Input: part model. Units: mm. Frame: model coordinates. Coordinates: 2 decimals unless noted, no trailing zeros. Order: outer loops, then holes, each group sorted by start corner. A loop starts at its lowest first (then second) coordinate and runs counter-clockwise, first axis right, second up. Notation, with made-up numbers: (-32.75, -39) -> (17.25, -39) arc R13 ccw to (17.25, -29) -> close; hole circle Ø2 at (41.25, -7). An arc over 180 degrees is marked (long way). Answer as CSV lines item,"result".
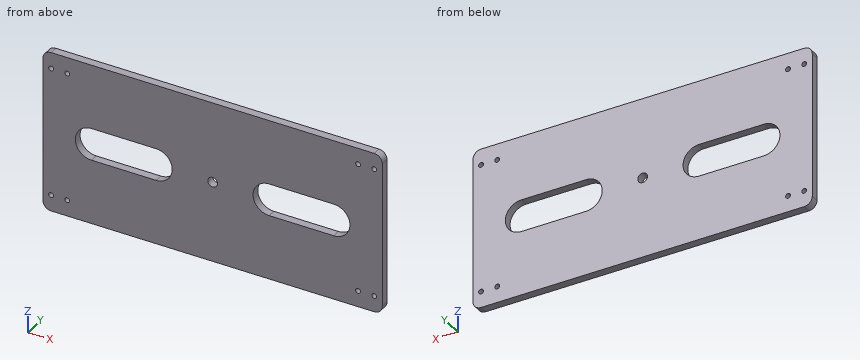
from build123d import *

# Parameters (mm, degrees)
SKETCH_1_W          = 210
SKETCH_1_H          = 100
EXTRUDE_1_DEPTH     = 5
CUT_EXTRUDE_1_DEPTH = 40
SKETCH_4_R          = 3
CUT_EXTRUDE_3_DEPTH = 20
SKETCH_8_R          = 1.5
CUT_EXTRUDE_4_DEPTH = 20
FILLET_1_R          = 5


with BuildPart() as part:
    # 草图1 → 凸台-拉伸1 (new body)
    with BuildSketch(Plane(origin=(0, 0, 0), x_dir=(1, 0, 0), z_dir=(0, 1, 0))):
        with Locations((105, -50)):
            Rectangle(SKETCH_1_W, SKETCH_1_H)
    extrude(amount=EXTRUDE_1_DEPTH)

    # 草图2 → 切除-拉伸1 (cut)
    with BuildSketch(Plane(origin=(0, 5, 0), x_dir=(1, 0, 0), z_dir=(0, 1, 0))):
        with BuildLine():
            Line((30, -40), (70, -40))
            ThreePointArc((70, -40), (80, -50), (70, -60))
            Line((70, -60), (30, -60))
            ThreePointArc((30, -60), (20, -50), (30, -40))
        make_face()
        with BuildLine():
            Line((140, -40), (180, -40))
            ThreePointArc((180, -40), (190, -50), (180, -60))
            Line((180, -60), (140, -60))
            ThreePointArc((140, -60), (130, -50), (140, -40))
        make_face()
    extrude(amount=-CUT_EXTRUDE_1_DEPTH, mode=Mode.SUBTRACT)

    # 草图4 → 切除-拉伸3 (cut)
    with BuildSketch(Plane(origin=(0, 5, 0), x_dir=(1, 0, 0), z_dir=(0, 1, 0))):
        with Locations(Location((105, -50, 0), (0, 0, 270))):
            Circle(SKETCH_4_R)
    extrude(amount=-CUT_EXTRUDE_3_DEPTH, mode=Mode.SUBTRACT)

    # 草图8 → 切除-拉伸4 (cut)
    with BuildSketch(Plane(origin=(0, 5, 0), x_dir=(1, 0, 0), z_dir=(0, 1, 0))):
        with Locations(Location((5, -10, 0), (0, 0, 270))):
            Circle(SKETCH_8_R)
        with Locations(Location((205, -10, 0), (0, 0, 270))):
            Circle(SKETCH_8_R)
        with Locations(Location((205, -90, 0), (0, 0, 270))):
            Circle(SKETCH_8_R)
        with Locations(Location((5, -90, 0), (0, 0, 270))):
            Circle(SKETCH_8_R)
        with Locations(Location((15, -10, 0), (0, 0, 270))):
            Circle(SKETCH_8_R)
        with Locations(Location((15, -90, 0), (0, 0, 270))):
            Circle(SKETCH_8_R)
        with Locations(Location((195, -90, 0), (0, 0, 270))):
            Circle(SKETCH_8_R)
        with Locations(Location((195, -10, 0), (0, 0, 270))):
            Circle(SKETCH_8_R)
    extrude(amount=-CUT_EXTRUDE_4_DEPTH, mode=Mode.SUBTRACT)

    # 圆角1
    fillet_1_edges = [part.edges().sort_by_distance(p)[0] for p in [
        (0, 2.5, 0),
        (210, 2.5, 0),
        (210, 2.5, 100),
        (0, 2.5, 100),
    ]]
    fillet(fillet_1_edges, radius=FILLET_1_R)


solid = part.part
1. Contact query for a flat-ended pin moving along its axis: pin 1 (1.8 mm diameter, centred on x = 15, z = 90, fed in from +Y). Output: stop coordinate, or through.
Findings:
pin 1,"passes through"
2. Cut plane B-B (y = 4.15). State how many separate pieces and enclosed holes the cut face has, plus the area to 3 significant figures.
Findings:
separate pieces,"1"
enclosed holes,"11"
area,"18,700 mm2"
3. Cut plane C-C (x = 185). Return the cut outline in (y, z), plus the area to 3 significant figures.
Findings:
outline,"(0, 0) -> (5, 0) -> (5, 41.34) -> (0, 41.34) -> close; (0, 58.66) -> (5, 58.66) -> (5, 100) -> (0, 100) -> close"
area,"413 mm2"
4. Cut plane A-A (x = 145). Return the cut outline in (y, z).
Findings:
outline,"(0, 0) -> (5, 0) -> (5, 40) -> (0, 40) -> close; (0, 60) -> (5, 60) -> (5, 100) -> (0, 100) -> close"
5. Ray query, line 1 along X through (y, z) = (3.7, 10); line 2 along Z through (x, y) = (195, 1.7); line 3 along Z through (x, y) = (45, 2.85). Return the intervals inside material, ascending.
Findings:
line 1,"x = 0 to 3.5, 6.5 to 13.5, 16.5 to 193.5, 196.5 to 203.5, 206.5 to 210"
line 2,"z = 0 to 8.5, 11.5 to 88.5, 91.5 to 100"
line 3,"z = 0 to 40, 60 to 100"
